Verification items for the finished model (mm, model axes). Give positions to 0.01 mm unless a question says otherwise; leave off trailing zeros. Order: outer loops, then holes, each group sorted by start corner. A loop starts at its lowest first (then second) coordinate and runs counter-clockwise, first axis right, second up.
from build123d import *

# Parameters (mm, degrees)
F0_R            = 50.3734102362
F1_DEPTH        = 25.4
F2_R            = 7.9966512346
F3_DEPTH        = 25.4
F3_COPIES_COUNT = 9


# Not quite as in the source:
# - a pattern or mirror of a feature is missing from the dataset's text; its kind, count and spacing are read off the source's solid


with BuildPart() as f1:
    # F0 (on Right) → F1 (new body)
    with BuildSketch(Plane.YZ):
        Circle(F0_R)
    extrude(amount=F1_DEPTH)

    # F2 (on face) → F3 (cut)
    with BuildSketch(Plane.YZ.offset(25.4)):
        with Locations((0, -24.4634896517)):
            Circle(F2_R)
    f3 = extrude(amount=-F3_DEPTH, mode=Mode.SUBTRACT)

    # F3_copies: F3 ×9 about axis
    f3_copies_axis = Axis((0, 0, 0), (1, 0, 0))
    for i in range(1, F3_COPIES_COUNT):
        add(f3.rotate(f3_copies_axis, i * 360 / F3_COPIES_COUNT), mode=Mode.SUBTRACT)


solid = f1.part
(1) Section check A-A, the plane z = 6.5. Enter the section's corners in (x, y).
Solved:
outline: (0, -49.95) - (25.4, -49.95) - (25.4, -26.76) - (0, -26.76) - close; (0, -15.61) - (25.4, -15.61) - (25.4, 15.61) - (0, 15.61) - close; (0, 26.76) - (25.4, 26.76) - (25.4, 49.95) - (0, 49.95) - close
(2) Release check for a two-part mould opening along Z. For faces 1 (the cylindrical face through (12.522, -50.325, 2.215)), 2 (the cylindrical face through (12.88, -13.8, 9.17)), 3 (the flat face through (25.4, -1, 1)) record: pulls with the +Z half, pulls with the -Z half, needs draft (parallel to the pull), parting line crosses it, or undercut.
Solved:
face 1: parting line crosses it
face 2: undercut
face 3: needs draft
(3) Section check D-D, the plane y = -36. Enter the section's corners in (x, z), then the cut area to 3 significant figures.
Solved:
outline: (0, -35.23) - (25.4, -35.23) - (25.4, 35.23) - (0, 35.23) - close
area: 1,790 mm2
(4) Go/stop test with flat-tipped pins: pin 1 (5 mm diameter, centred on y = -17.5, z = -35, fed in from -X); pin 2 (13 mm diameter, centred on y = 8.37, z = 22.99, fed in from -X); pin 3 (3 mm diameter, centred on x = 13, z = 27.5, fed in from +Y); pin 4 (1.5 mm diameter, centred on x = 8.5, y = -27, fed in from -Z). Record where each tip stops, or that it passes through.
Solved:
pin 1: stops at x = 0
pin 2: passes through
pin 3: stops at y = 43.14
pin 4: stops at z = -42.99
(5) Scan lines: line 1 (Y direction, x = 7.75, z = -25); line 2 (Y direction, x = 19.75, z = -15); line 3 (Y direction, x = 5, z = 18). Record each from-to range of solid material in increasing order.
Solved:
line 1: y = -43.73 to -20.7, -10.75 to -7.98, 7.98 to 10.75, 20.7 to 43.73
line 2: y = -48.09 to -22.79, -8.66 to 8.66, 22.79 to 48.09
line 3: y = -47.05 to -26.72, -15.65 to -14.62, -2.12 to 2.12, 14.62 to 15.65, 26.72 to 47.05
(6) Section check C-C, the plane z = 28. Enter the section's corners in (x, y).
Solved:
outline: (0, -41.87) - (25.4, -41.87) - (25.4, -14.6) - (0, -14.6) - close; (0, -2.14) - (25.4, -2.14) - (25.4, 2.14) - (0, 2.14) - close; (0, 14.6) - (25.4, 14.6) - (25.4, 41.87) - (0, 41.87) - close
(7) Section check B-B, the plane x = 14. Give the number of separate pieces and of enclosed holes in the cut face, then the cut area to 3 significant figures.
Solved:
separate pieces: 1
enclosed holes: 9
area: 6,160 mm2
